Read the model definition and answer for the solid it produces. Units are mm, in the model's axes. Face numbers are marked on the shaded views. A direction names the side the tool comes from. Coordinates: 2 decimals unless noted, no trailing zeros. Loops run counter-clockwise (first coordinate to the right, second up) from the corner with the lowest first, then second, coordinate; pieces in that order, holes last.
Q1. Section D-D (z = -11) is taken. Give the vertices of the cut face in (x, y), then the cut area to 3 significant figures.
Q2. Straight lines are drawn through the part: line 1 (Z direction, x = 56, y = 7.65); line 2 (X direction, y = 5.25, z = -21); line 3 (X direction, y = 5.5, z = -5). For each, find the intervals that lie inside material, in ascending order.
Q3. Which of the six approach directions +Z, -Z, +X, -X, +Y, -Y give full straight-line access (tool end or side, diameter ignored) to the marked faces 1, 2 and 3?
Q4. Section C-C (x = 16) is taken. Give the vertices of the cut face in (y, z).
Q5. Section A-A (x = 136) is taken. Give the vertices of the cut face in (y, z).
Q6. Section B-B (z = -40) is taken. Give the vertices of the cut face in (x, y), then the cut area to 3 significant figures.
Q7. Flat-ended cylindrical pins translate along their axes: P1, Ø4.5, axis at x = 96.5, z = -65, coming from the +Y side; P2, Ø4, axis at x = 145.96, z = -55.5, coming from the -Y side; P3, Ø5.5, axis at x = 37.5, z = -31, coming from the +Y side. Find the tip coordinate at first contact, or state that the pin passes through.
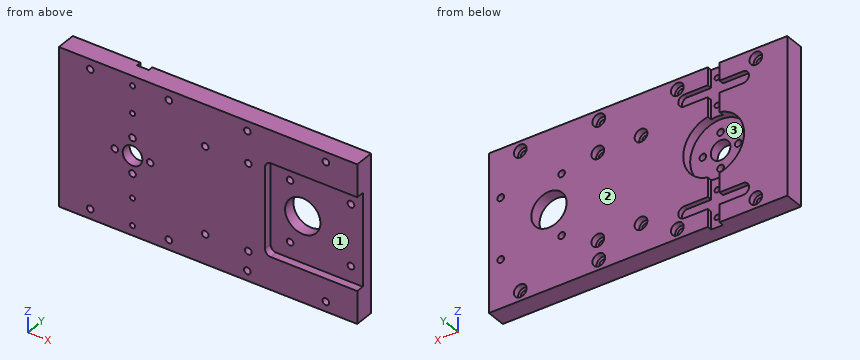
from build123d import *

# Parameters (mm, degrees)
SKETCH1_W                                = 152
SKETCH1_H                                = 80
BOSS_EXTRUDE1_DEPTH                      = 10
SKETCH2_R                                = 15.5
CUT_EXTRUDE1_DEPTH                       = 5
SKETCH3_R                                = 5
CUT_EXTRUDE2_DEPTH                       = 5
CUT_EXTRUDE3_DEPTH                       = 2.5
CIRPATTERN1_COUNT                        = 2
SKETCH5_R                                = 9
CUT_EXTRUDE4_DEPTH                       = 6
SKETCH6_W                                = 47
SKETCH6_H                                = 47
CUT_EXTRUDE5_DEPTH                       = 4
FILLET1_R                                = 3
CBORE_FOR_M3_PAN_HEAD_SCREW1_D           = 3.4
CBORE_FOR_M3_PAN_HEAD_SCREW1_CBORE_D     = 6.5
CBORE_FOR_M3_PAN_HEAD_SCREW1_CBORE_DEPTH = 3
CBORE_FOR_M3_PAN_HEAD_SCREW2_D           = 3.4
CBORE_FOR_M3_PAN_HEAD_SCREW2_CBORE_D     = 6.5
CBORE_FOR_M3_PAN_HEAD_SCREW2_CBORE_DEPTH = 3.3
TAP_DRILL_FOR_M3X0_5_TAP1_D              = 2.6
TAP_DRILL_FOR_M3X0_5_TAP2_D              = 3.4
TAP_DRILL_FOR_M3X0_5_TAP3_D              = 3.4


with BuildPart() as part:
    # Sketch1 → Boss-Extrude1 (new body)
    with BuildSketch(Plane(origin=(0, 0, 0), x_dir=(1, 0, 0), z_dir=(0, 1, 0))):
        with Locations((76, 40)):
            Rectangle(SKETCH1_W, SKETCH1_H)
    extrude(amount=BOSS_EXTRUDE1_DEPTH)

    # Sketch2 → Cut-Extrude1 (cut)
    with BuildSketch(Plane(origin=(0, 10, 0), x_dir=(1, 0, 0), z_dir=(0, 1, 0))):
        with Locations(Location((37.5, 40, 0), (0, 0, 270))):
            Circle(SKETCH2_R)
    extrude(amount=-CUT_EXTRUDE1_DEPTH, mode=Mode.SUBTRACT)

    # Sketch3 → Cut-Extrude2 (cut)
    with BuildSketch(Plane(origin=(0, 5, 0), x_dir=(1, 0, 0), z_dir=(0, 1, 0))):
        with Locations(Location((37.5, 40, 0), (0, 0, 270))):
            Circle(SKETCH3_R)
    extrude(amount=-CUT_EXTRUDE2_DEPTH, mode=Mode.SUBTRACT)

    # Sketch4 → Cut-Extrude3 (cut)
    with BuildSketch(Plane(origin=(0, 10, 0), x_dir=(1, 0, 0), z_dir=(0, 1, 0))):
        with BuildLine():
            Line((34.5, 24.793093674), (34.5, 15))
            Line((34.5, 15), (22.5, 15))
            ThreePointArc((22.5, 15), (19.5, 12), (22.5, 9))
            Line((22.5, 9), (34.5, 9))
            Line((34.5, 9), (34.5, 0))
            Line((34.5, 0), (40.5, 0))
            Line((40.5, 0), (40.5, 9))
            Line((40.5, 9), (52.5, 9))
            ThreePointArc((52.5, 9), (55.5, 12), (52.5, 15))
            Line((52.5, 15), (40.5, 15))
            Line((40.5, 15), (40.5, 24.793093674))
            ThreePointArc((40.5, 24.793093674), (37.5, 24.5), (34.5, 24.793093674))
        make_face()
    cut_extrude3 = extrude(amount=-CUT_EXTRUDE3_DEPTH, mode=Mode.SUBTRACT)

    # CirPattern1: Cut-Extrude3 ×2 about axis
    cirpattern1_axis = Axis((37.5, 0, -40), (0, 1, 0))
    for i in range(1, CIRPATTERN1_COUNT):
        add(cut_extrude3.rotate(cirpattern1_axis, i * 360 / CIRPATTERN1_COUNT), mode=Mode.SUBTRACT)

    # Sketch5 → Cut-Extrude4 (cut)
    with BuildSketch(Plane(origin=(0, 10, 0), x_dir=(1, 0, 0), z_dir=(0, 1, 0))):
        with Locations(Location((121.41, 40, 0), (0, 0, 270))):
            Circle(SKETCH5_R)
    extrude(amount=-CUT_EXTRUDE4_DEPTH, mode=Mode.SUBTRACT)

    # Sketch6 → Cut-Extrude5 (cut)
    with BuildSketch(Plane(origin=(0, 4, 0), x_dir=(1, 0, 0), z_dir=(0, 1, 0))):
        with Locations((128.5, 40)):
            Rectangle(SKETCH6_W, SKETCH6_H)
    extrude(amount=-CUT_EXTRUDE5_DEPTH, mode=Mode.SUBTRACT)

    # Fillet1
    fillet1_edges = [part.edges().sort_by_distance(p)[0] for p in [
        (105, 2, -16.5),
        (105, 2, -63.5),
    ]]
    fillet(fillet1_edges, radius=FILLET1_R)

    # CBORE for M3 Pan Head Screw1 (through all)
    with Locations(Plane(origin=(0, 10, 0), x_dir=(1, 0, 0), z_dir=(0, 1, 0))):
        with Locations((16, 75), (56, 75), (16, 5), (56, 5), (96, 75), (96, 5), (136, 5), (136, 75)):
            CounterBoreHole(CBORE_FOR_M3_PAN_HEAD_SCREW1_D / 2, CBORE_FOR_M3_PAN_HEAD_SCREW1_CBORE_D / 2, CBORE_FOR_M3_PAN_HEAD_SCREW1_CBORE_DEPTH)

    # CBORE for M3 Pan Head Screw2 (through all)
    with Locations(Plane(origin=(0, 10, 0), x_dir=(1, 0, 0), z_dir=(0, 1, 0))):
        with Locations((96.5, 65), (96.5, 21), (74.5, 21), (74.5, 65)):
            CounterBoreHole(CBORE_FOR_M3_PAN_HEAD_SCREW2_D / 2, CBORE_FOR_M3_PAN_HEAD_SCREW2_CBORE_D / 2, CBORE_FOR_M3_PAN_HEAD_SCREW2_CBORE_DEPTH)

    # Tap Drill for M3x0.5 Tap1 (through all)
    with Locations(Plane(origin=(0, 7.5, 0), x_dir=(1, 0, 0), z_dir=(0, 1, 0))):
        with Locations((37.5, 75), (37.5, 61.2), (37.5, 18.8), (37.5, 5)):
            Hole(TAP_DRILL_FOR_M3X0_5_TAP1_D / 2)

    # Tap Drill for M3x0.5 Tap2 (through all)
    with Locations(Plane(origin=(0, 10, 0), x_dir=(1, 0, 0), z_dir=(0, 1, 0))):
        with Locations((114.96, 55.5), (145.96, 55.5), (114.96, 24.5), (145.96, 24.5)):
            Hole(TAP_DRILL_FOR_M3X0_5_TAP2_D / 2)

    # Tap Drill for M3x0.5 Tap3 (through all)
    with Locations(Plane(origin=(0, 5, 0), x_dir=(1, 0, 0), z_dir=(0, 1, 0))):
        with Locations((37.5, 49), (46.5, 40), (28.5, 40), (37.5, 31)):
            Hole(TAP_DRILL_FOR_M3X0_5_TAP3_D / 2)


solid = part.part
Numbers:
1. outline: (0, 0) - (152, 0) - (152, 10) - (55.33, 10) - (55.33, 7.5) - (19.67, 7.5) - (19.67, 10) - (0, 10) - close
1. area: 1,430 mm2
2. line 1: z = -80 to -78.25, -71.75 to -8.25, -1.75 to 0
2. line 2: x = 0 to 72.8, 76.2 to 94.8, 98.2 to 152
2. line 3: x = 0 to 14.3, 17.7 to 36.2, 38.8 to 54.3, 57.7 to 94.3, 97.7 to 134.3, 137.7 to 152
3. face 1: +X, -Y
3. face 2: +Z, -Z, +X, -X, +Y
3. face 3: +Y
4. outline: (0, -80) - (10, -80) - (10, -78.25) - (7, -78.25) - (7, -76.7) - (0, -76.7) - close; (0, -73.3) - (7, -73.3) - (7, -71.75) - (10, -71.75) - (10, -8.25) - (7, -8.25) - (7, -6.7) - (0, -6.7) - close; (0, -3.3) - (7, -3.3) - (7, -1.75) - (10, -1.75) - (10, 0) - (0, 0) - close
5. outline: (0, -80) - (10, -80) - (10, -78.25) - (7, -78.25) - (7, -76.7) - (0, -76.7) - close; (0, -73.3) - (7, -73.3) - (7, -71.75) - (10, -71.75) - (10, -8.25) - (7, -8.25) - (7, -6.7) - (0, -6.7) - (0, -16.5) - (4, -16.5) - (4, -63.5) - (0, -63.5) - close; (0, -3.3) - (7, -3.3) - (7, -1.75) - (10, -1.75) - (10, 0) - (0, 0) - close
6. outline: (0, 0) - (26.8, 0) - (26.8, 5) - (22, 5) - (22, 10) - (0, 10) - close; (30.2, 0) - (32.5, 0) - (32.5, 5) - (30.2, 5) - close; (42.5, 0) - (44.8, 0) - (44.8, 5) - (42.5, 5) - close; (48.2, 0) - (105, 0) - (105, 4) - (112.41, 4) - (112.41, 10) - (53, 10) - (53, 5) - (48.2, 5) - close; (130.41, 4) - (152, 4) - (152, 10) - (130.41, 10) - close
6. area: 985 mm2
7. P1: stops at y = 6.7
7. P2: stops at y = 4
7. P3: stops at y = 5
